from build123d import *

# Parameters (mm, degrees)
SKETCH_1_W          = 10.5
SKETCH_1_H          = 1.3
EXTRUDE_1_DEPTH     = 10
SKETCH_2_R          = 3
CUT_EXTRUDE_1_DEPTH = 5
SKETCH_3_R          = 3
EXTRUDE_2_DEPTH     = 10
SKETCH_4_R          = 1.7
EXTRUDE_3_DEPTH     = 5
SKETCH_5_R          = 1.5
CUT_EXTRUDE_2_DEPTH = 5
FILLET_1_R          = 1


with BuildPart() as part:
    # 草图1 → 凸台-拉伸1 (new body, symmetric)
    with BuildSketch(Plane(origin=(0, 0, 0), x_dir=(0, 0, -1), z_dir=(1, 0, 0))):
        with Locations((5.25, 0.65)):
            Rectangle(SKETCH_1_W, SKETCH_1_H)
    extrude(amount=EXTRUDE_1_DEPTH, both=True)

    # 草图2 → 切除-拉伸1 (cut)
    with BuildSketch(Plane(origin=(10, 0, 0), x_dir=(0, 0, -1), z_dir=(1, 0, 0))):
        with Locations((0, 3)):
            Circle(SKETCH_2_R)
    cut_extrude_1 = extrude(amount=-CUT_EXTRUDE_1_DEPTH, mode=Mode.SUBTRACT)

    # 草图3 → 凸台-拉伸2 (add)
    with BuildSketch(Plane(origin=(5, 0, 0), x_dir=(0, 0, -1), z_dir=(1, 0, 0))):
        with Locations((0, 3)):
            Circle(SKETCH_3_R)
    extrude(amount=-EXTRUDE_2_DEPTH)

    # 草图4 → 凸台-拉伸3 (add)
    with BuildSketch(Plane(origin=(5, 0, 0), x_dir=(0, 0, -1), z_dir=(1, 0, 0))):
        with Locations((0, 3)):
            Circle(SKETCH_4_R)
    extrude_3 = extrude(amount=EXTRUDE_3_DEPTH)

    # 镜向1: 切除-拉伸1, 凸台-拉伸3 across plane
    add(cut_extrude_1.mirror(Plane(origin=(0, 0, 0), x_dir=(0, 0, 1), z_dir=(1, 0, 0))), mode=Mode.SUBTRACT)
    add(extrude_3.mirror(Plane(origin=(0, 0, 0), x_dir=(0, 0, 1), z_dir=(1, 0, 0))))

    # 草图5 → 切除-拉伸2 (cut)
    with BuildSketch(Plane(origin=(0, 1.3, 0), x_dir=(1, 0, 0), z_dir=(0, 1, 0))):
        with Locations((-6, 7.5)):
            Circle(SKETCH_5_R)
    cut_extrude_2 = extrude(amount=-CUT_EXTRUDE_2_DEPTH, mode=Mode.SUBTRACT)

    # 镜向2: 切除-拉伸2 across plane
    add(cut_extrude_2.mirror(Plane(origin=(0, 0, 0), x_dir=(0, 0, 1), z_dir=(1, 0, 0))), mode=Mode.SUBTRACT)

    # 圆角1
    fillet_1_edges = [part.edges().sort_by_distance(p)[0] for p in [
        (10, 0.65, -10.5),
        (-10, 0.65, -10.5),
    ]]
    fillet(fillet_1_edges, radius=FILLET_1_R)


solid = part.part
The model under review builds one solid part; all positions refer to its coordinate system, in mm. A direction names the side the tool comes from. Coordinates: 2 decimals unless noted, no trailing zeros. Loops run counter-clockwise (first coordinate to the right, second up) from the corner with the lowest first, then second, coordinate; pieces in that order, holes last. Notation, with made-up numbers: (-15.5, 44.5) -> (9.5, 44.5) arc R4 cw to (9.5, 48.5) -> close; hole circle Ø10 at (52.5, 2). An arc over 180 degrees is marked (long way). Use a Markdown table: item, result. Add a question column.
1. Add section B-B on z = -7.5. Write out the cut boundary in (x, y), plus the area to 3 significant figures.
2. Machinability: for faces 1 (the face through (5, 3, -2)), 2 (the face through (0.07, 5.705, 1.297)), 3 (the face through (-5, 3, -2)), which of the approach directions +Z, -Z, +X, -X, +Y, -Y give a long, thin tool a straight path to every point of the face, cutting with its end or side? Answer none if there is none.
3. Draft analysis for pull direction Y (two halves, no side actions). For faces 4 (the face through (-7.535, 0.335, -1.378)), 5 (the face through (10, 1, -6)), 6 (the face through (0, 0, -5)), state which applies: pulls with the +Y half, pulls with the -Y half, needs draft (parallel to the pull), parting line crosses it, or undercut.
4. To check wall thickness, follow line 1 (X direction, y = 0.4, z = -7.5); line 2 (X direction, y = 1.15, z = -8.25); line 3 (Y direction, x = 4.5, z = -9). State the ranges of each line that lie inside material, in increasing order.
5. Add section A-A on x = 6. Write out the cut boundary in (y, z).
6. Clearance check with flat-ended pins moving along their axes: pin 1 Ø3 at (x, z) = (-5.5, -7) entering from +Y; pin 2 Ø3 at (x, y) = (0.5, 3) entering from -Z; pin 3 Ø2 at (x, z) = (-7, -6) entering from -Y; pin 4 Ø1.8 at (x, z) = (-6, -7.5) entering from -Y. State where each tip first meets the part, or that it passes through.
7. Add section C-C on y = 3. Write out the cut boundary in (x, z).
8. Add section D-D on y = 1.05. Write out the cut boundary in (x, z).
Returned:
| question | item | result |
|---|---|---|
| 1 | outline | (-10, 0) -> (-7.5, 0) -> (-7.5, 1.3) -> (-10, 1.3) -> close; (-4.5, 0) -> (4.5, 0) -> (4.5, 1.3) -> (-4.5, 1.3) -> close; (7.5, 0) -> (10, 0) -> (10, 1.3) -> (7.5, 1.3) -> close |
| 1 | area | 18.2 mm² |
| 2 | face 1 | +X |
| 2 | face 2 | +X, -X |
| 2 | face 3 | -X |
| 3 | face 4 | undercut |
| 3 | face 5 | needs draft |
| 3 | face 6 | pulls with the -Y half |
| 4 | line 1 | x = -10 to -7.5, -4.5 to 4.5, 7.5 to 10 |
| 4 | line 2 | x = -10 to -7.3, -4.7 to 4.7, 7.3 to 10 |
| 4 | line 3 | y = 0 to 1.3 |
| 5 | outline | (0, -10.5) -> (1.3, -10.5) -> (1.3, -9) -> (0, -9) -> close; (0, -6) -> (1.3, -6) -> (1.3, -2.47) arc R3 cw to (0, 0) -> close; circle Ø3.4 at (3, 0) |
| 6 | pin 1 | stops at y = 1.3 |
| 6 | pin 2 | stops at z = -3 |
| 6 | pin 3 | stops at y = 0 |
| 6 | pin 4 | passes through |
| 7 | outline | (-10, -1.7) -> (-5, -1.7) -> (-5, -3) -> (5, -3) -> (5, -1.7) -> (10, -1.7) -> (10, 1.7) -> (5, 1.7) -> (5, 3) -> (-5, 3) -> (-5, 1.7) -> (-10, 1.7) -> close |
| 8 | outline | (-10, -9.5) arc R1 ccw to (-9, -10.5) -> (9, -10.5) arc R1 ccw to (10, -9.5) -> (10, -2.28) -> (5, -2.28) -> (5, 2.28) -> (-5, 2.28) -> (-5, -2.28) -> (-10, -2.28) -> close; hole circle Ø3 at (-6, -7.5); hole circle Ø3 at (6, -7.5) |
